from build123d import *

# Parameters (mm, degrees)
EXTRUDE_1_DEPTH          = 7
EXTRUDE_1_DEPTH_BACK     = 2.4
SKETCH_1_W               = 60.5
SKETCH_1_H               = 60.5
SKETCH_1_W_2             = 38.5
SKETCH_1_H_2             = 38.5
SKETCH_2_W               = 38.5
SKETCH_2_H               = 38.5
SKETCH_2_W_2             = 25
SKETCH_2_H_2             = 25
EXTRUDE_3_DEPTH          = 5.8
CUT_EXTRUDE_1_DEPTH      = 2.4
CUT_EXTRUDE_2_DEPTH      = 44.800513696
CUT_EXTRUDE_2_DEPTH_BACK = 44.800513696
SKETCH_5_R               = 1.6


with BuildPart() as part:
    # ｽｹｯﾁ1 → ﾎﾞｽ - 押し出し1 (new, two sides: drawn at the far end of the back side and taken through both)
    with BuildSketch(Plane.XY.offset(-EXTRUDE_1_DEPTH_BACK)):
        Rectangle(SKETCH_1_W, SKETCH_1_H)
        Rectangle(SKETCH_1_W_2, SKETCH_1_H_2, mode=Mode.SUBTRACT)
    extrude(amount=EXTRUDE_1_DEPTH + EXTRUDE_1_DEPTH_BACK)

    # ｽｹｯﾁ2 → ﾎﾞｽ - 押し出し3 (add)
    with BuildSketch(Plane.XY.offset(1.2)):
        Rectangle(SKETCH_2_W, SKETCH_2_H)
        Rectangle(SKETCH_2_W_2, SKETCH_2_H_2, mode=Mode.SUBTRACT)
    extrude(amount=EXTRUDE_3_DEPTH)

    # ｽｹｯﾁ3 → ｶｯﾄ - 押し出し1 (cut)
    with BuildSketch(Plane(origin=(0, 0, -2.4), x_dir=(-1, 0, 0), z_dir=(0, 0, -1))):
        with BuildLine():
            ThreePointArc((-24.95, 19.25), (-23.280508653, 23.280508653), (-19.25, 24.95))
            Line((-19.25, 24.95), (19.25, 24.95))
            ThreePointArc((19.25, 24.95), (23.280508653, 23.280508653), (24.95, 19.25))
            Line((24.95, 19.25), (24.95, -19.25))
            ThreePointArc((24.95, -19.25), (23.280508653, -23.280508653), (19.25, -24.95))
            Line((19.25, -24.95), (-19.25, -24.95))
            ThreePointArc((-19.25, -24.95), (-23.280508653, -23.280508653), (-24.95, -19.25))
            Line((-24.95, -19.25), (-24.95, 19.25))
        make_face()
        with BuildLine():
            Line((-20.75, -19.25), (-20.75, 19.25))
            ThreePointArc((-20.75, 19.25), (-20.310660172, 20.310660172), (-19.25, 20.75))
            Line((-19.25, 20.75), (19.25, 20.75))
            ThreePointArc((19.25, 20.75), (20.310660172, 20.310660172), (20.75, 19.25))
            Line((20.75, 19.25), (20.75, -19.25))
            ThreePointArc((20.75, -19.25), (20.310660172, -20.310660172), (19.25, -20.75))
            Line((19.25, -20.75), (-19.25, -20.75))
            ThreePointArc((-19.25, -20.75), (-20.310660172, -20.310660172), (-20.75, -19.25))
        make_face(mode=Mode.SUBTRACT)
    extrude(amount=-CUT_EXTRUDE_1_DEPTH, mode=Mode.SUBTRACT)

    # ｽｹｯﾁ5 → ｶｯﾄ - 押し出し2 (cut, two sides: drawn at the far end of the back side and taken through both)
    with BuildSketch(Plane(origin=(0, 0, -2.4), x_dir=(-1, 0, 0), z_dir=(0, 0, -1)).offset(-CUT_EXTRUDE_2_DEPTH_BACK)):
        with Locations((-25.75, 25.75)):
            Circle(SKETCH_5_R)
        with Locations((25.75, 25.75)):
            Circle(SKETCH_5_R)
        with Locations((25.75, -25.75)):
            Circle(SKETCH_5_R)
        with Locations((-25.75, -25.75)):
            Circle(SKETCH_5_R)
    extrude(amount=CUT_EXTRUDE_2_DEPTH + CUT_EXTRUDE_2_DEPTH_BACK, mode=Mode.SUBTRACT)


solid = part.part
Design review of the part built by this model. Coordinates are the model's own, in mm. A direction names the side the tool comes from. Coordinates: 2 decimals unless noted, no trailing zeros. Order: outer loops, then holes, each group sorted by start corner. A loop starts at its lowest first (then second) coordinate and runs counter-clockwise, first axis right, second up. Notation, with made-up numbers: (-6, 74) -> (25, 74) arc R23 cw to (25, 111) -> close; hole circle Ø11 at (22.25, -34.75). An arc over 180 degrees is marked (long way). One line per item, written item: value.
1) To check wall thickness, follow probe 1 along Y at (x, z) = (-25.75, 0.5); probe 2 along X at (y, z) = (7.5, -1.75). State the ranges of each line that lie inside material, in increasing order. Write a range as [from, to].
Output values:
probe 1: y = [-30.25, -27.35], [-24.15, 24.15], [27.35, 30.25]
probe 2: x = [-30.25, -24.95], [-20.75, -19.25], [19.25, 20.75], [24.95, 30.25]
2) Clearance check with flat-ended pins moving along their axes: P1, Ø2.5, axis at x = -25.75, y = -25.75, coming from the +Z side; P2, Ø15, axis at x = -11, y = -2.5, coming from the -Z side; P3, Ø4, axis at x = -25.75, y = 25.75, coming from the +Z side. State where each tip first meets the part, or that it passes through.
Output values:
P1: passes through
P2: stops at z = 1.2
P3: stops at z = 7
3) We need section B-B, the plane y = -3.5. Give the boundary of the cut face in (x, z), then the cut area to 3 significant figures.
Output values:
outline: (-30.25, -2.4) -> (-24.95, -2.4) -> (-24.95, 0) -> (-20.75, 0) -> (-20.75, -2.4) -> (-19.25, -2.4) -> (-19.25, 1.2) -> (-12.5, 1.2) -> (-12.5, 7) -> (-30.25, 7) -> close; (12.5, 1.2) -> (19.25, 1.2) -> (19.25, -2.4) -> (20.75, -2.4) -> (20.75, 0) -> (24.95, 0) -> (24.95, -2.4) -> (30.25, -2.4) -> (30.25, 7) -> (12.5, 7) -> close
area: 265 mm2
4) Draft analysis for pull direction Y (two halves, no side actions). For faces 1 (the face through (-20.75, 0, -1)), 2 (the face through (-30.25, 0, 2)), state which applies: +Y half, -Y half, draft (parallel to the pull), parting line (faces both ways), or undercut.
Output values:
face 1: undercut
face 2: draft
5) We need section A-A, the plane x = 25.75. Give the boundary of the cut face in (y, z).
Output values:
outline: (-30.25, -2.4) -> (-27.35, -2.4) -> (-27.35, 7) -> (-30.25, 7) -> close; (-24.15, -2.4) -> (24.15, -2.4) -> (24.15, 7) -> (-24.15, 7) -> close; (27.35, -2.4) -> (30.25, -2.4) -> (30.25, 7) -> (27.35, 7) -> close
6) Machinability: for faces 3 (the face through (22, 0, 0)), 4 (the face through (-12.5, 0, 4)), 5 (the face through (-14, 0, 7)), which of the approach directions +Z, -Z, +X, -X, +Y, -Y give a long, thin tool a straight path to every point of the face, cutting with its end or side? Answer none if there is none.
Output values:
face 3: -Z
face 4: +Z, -Z
face 5: +Z, +X, -X, +Y, -Y
